Source: CAD feature listing. Evaluate the final solid. Frame: model axes, mm. A direction names the side the tool comes from. Round coordinates to 2 decimals unless told otherwise and drop trailing zeros. Write each loop counter-clockwise with the first axis right and the second up, starting at its lowest first coordinate (ties: lowest second). Pieces come first, ordered by that corner, then holes.
Autodesk Inventor part; units mm, degrees
ref_plane "YZ Plane" through (0, 0, 0) normal (1, 0, 0) x (0, 1, 0)
ref_plane "XZ Plane" through (0, 0, 0) normal (0, 1, 0) x (-1, 0, 0)
ref_plane "XY Plane" through (0, 0, 0) normal (0, 0, 1) x (1, 0, 0)
sketch "Sketch1" plane through (0, 0, 0) normal (0, 0, 1) x (1, 0, 0)
  line L0 (0, 0) -> (27, 0)
  line L1 (27, 0) -> (27, 10)
  line L2 (27, 10) -> (0, 10)
  line L3 (0, 10) -> (0, 0)
  line L4 (7.5, 0) -> (19.5, 0)
  line L5 (19.5, 0) -> (19.5, 5)
  line L6 (19.5, 5) -> (7.5, 5)
  line L7 (7.5, 5) -> (7.5, 0)
  point P0 (13.5, 5)
  point P1 (13.5, 10)
  dimension "d0" = 27
  dimension "d1" = 10
  dimension "d2" = 5
  dimension "d3" = 12
extrude "Extrusion1" add sketch "Sketch1" along normal blind 34.7 contours L3 L2 L1 L0 L5 L6 L7
chamfer "Chamfer1" distance 1 angle 45 2 edges at (27, 10, 17.35) (0, 10, 17.35)
chamfer "Chamfer2" distance 0.5 angle 45 2 edges at (7.5, 5, 17.35) (19.5, 5, 17.35)
sketch "Sketch2" plane through (1, 10, 0) normal (0, 1, 0) x (1, 0, 0)
  line L0 (18, -34.7) -> (18, 0)
  line L1 (-1, 0) -> (-1, -34.7)
  line L2 (25, 0) -> (0, 0)
  line L3 (5, -9.85) -> (20, -9.85)
  line L4 (20, -9.85) -> (20, -24.85)
  line L5 (20, -24.85) -> (5, -24.85)
  line L6 (5, -24.85) -> (5, -9.85)
  line L7 (25, 0) -> (25, -34.7)
  point P0 (-1, -17.35)
  point P1 (12.5, 0)
  point P2 (12.5, -9.85)
  point P3 (12.5, 0)
  point P4 (20, -17.35)
  point P5 (25, -17.35)
  dimension "d12" = 15
  dimension "d13" = 15
hole "Hole1" at (21, 10, 9.85) at (21, 10, 24.85) at (6, 10, 24.85) at (6, 10, 9.85) direction (0, -1, 0) diameter 3.242 depth 5 tip angle 118
sketch "Sketch3" plane through (0, 0, 34.7) normal (0, 0, 1) x (1, 0, 0)
  line L0 (0, 9) -> (0, 0)
  line L1 (0, 9) -> (1, 10)
  line L2 (26, 10) -> (1, 10)
  line L3 (26, 10) -> (27, 9)
  line L4 (27, 0) -> (27, 9)
  line L5 (0.375, 0) -> (0.375, 8.8447)
  line L6 (0.375, 8.8447) -> (1.1553, 9.625)
  line L7 (1.1553, 9.625) -> (25.8447, 9.625)
  line L8 (25.8447, 9.625) -> (26.625, 8.8447)
  line L9 (26.625, 8.8447) -> (26.625, 0)
  line L10 (19.5, 0) -> (27, 0)
  line L11 (26.625, 0) -> (27, 0)
  line L12 (27, 0) -> (0.375, 0)
  line L13 (0, 0) -> (7.5, 0)
  line L14 (0.375, 0) -> (0, 0)
  dimension "d21" = 0.375
extrude "Extrusion2" cut sketch "Sketch3" against normal blind 5 contours L1 L2 L3 L4 L10 L9 L8 L7 L6 L5 L13 L0
ref_plane "Work Plane1" through (0, 0, 17.35) normal (0, 0, 1) x (1, 0, 0)
mirror "Mirror1" about plane through (0, 0, 17.35) normal (0, 0, 1) of "Extrusion2"
sketch "Sketch4" plane through (1, 10, 29.7) normal (0, 1, 0) x (1, 0, 0)
  circle A0 centre (5, 19.85) radius 1.621
  circle A1 centre (20, 4.85) radius 1.621
  circle A2 centre (20, 19.85) radius 1.621
  circle A3 centre (5, 4.85) radius 1.621
  line L0 (25, 24.7) -> (0, 24.7)
  line L1 (0, 0) -> (0, 24.7)
  line L2 (0, 0) -> (25, 0)
  line L3 (25, 24.7) -> (25, 0)
  line L4 (25, 24.7) -> (0, 24.7)
  line L5 (0, 0) -> (25, 0)
  line L6 (9, 24.7) -> (16, 24.7)
  line L7 (16, 24.7) -> (16, 0)
  line L8 (16, 0) -> (9, 0)
  line L9 (9, 0) -> (9, 24.7)
  point P0 (-1, 29.7)
  point P1 (12.5, 24.7)
  point P2 (12.5, 24.7)
  dimension "d24" = 7
extrude "Extrusion3" cut sketch "Sketch4" against normal blind 0.35 contours L7 L2 L9 L0
properties part number "MGN Block"
1) Section query C-C on x = 15.25. Return the cut outline in (y, z) (3 decimals), then the cut area to 3 significant figures.
Taken from the geometry:
outline: (5, 0) - (9.625, 0) - (9.625, 5) - (9.65, 5) - (9.65, 29.7) - (9.625, 29.7) - (9.625, 34.7) - (5, 34.7) - close
area: 161 mm2
2) Section query A-A on y = 2.25. Return the cut outline in (x, z) (3 decimals).
Taken from the geometry:
outline: (0, 5) - (0.375, 5) - (0.375, 0) - (7.5, 0) - (7.5, 34.7) - (0.375, 34.7) - (0.375, 29.7) - (0, 29.7) - close; (19.5, 0) - (26.625, 0) - (26.625, 5) - (27, 5) - (27, 29.7) - (26.625, 29.7) - (26.625, 34.7) - (19.5, 34.7) - close
3) Material intervals for line 1 (Z direction, x = 6, y = 6.2); line 2 (X direction, y = 7.15, z = 9.85); line 3 (X direction, y = 4.5, z = 25), sorted ascending.
Taken from the geometry:
line 1: z = 0 to 8.23, 11.47 to 23.23, 26.47 to 34.7
line 2: x = 0 to 4.38, 7.62 to 19.38, 22.62 to 27
line 3: x = 0 to 5.23, 6.77 to 7.5, 19.5 to 20.23, 21.77 to 27
4) Section query B-B on z = 16. Return the cut outline in (x, y), then the cut area to 3 significant figures.
Taken from the geometry:
outline: (0, 0) - (7.5, 0) - (7.5, 4.5) - (8, 5) - (19, 5) - (19.5, 4.5) - (19.5, 0) - (27, 0) - (27, 9) - (26, 10) - (17, 10) - (17, 9.65) - (10, 9.65) - (10, 10) - (1, 10) - (0, 9) - close
area: 207 mm2
5) Contact query for flat-ended pins moving along their axis: P1, Ø1.5, axis at x = 18, z = 3, coming from the +Y side (3 decimals); P2, Ø5.5, axis at x = 16, z = 13.5, coming from the -Y side; P3, Ø2.5, axis at y = 4.5, z = 2.5, coming from the +X side (3 decimals). Output: stop coordinate, or through.
Taken from the geometry:
P1: stops at y = 9.625
P2: stops at y = 5
P3: stops at x = 26.625
6) Reachability of faces 4 (the face through (26.625, 4, 32)), 5 (the face through (14, 5, 17)), 6 (the face through (21.986, 7.465, 23.564)), 7 (the face through (14, 9.625, 2)), 8 (the face through (26.625, 4, 2)) from +Z, -Z, +X, -X, +Y, -Y: full face, straight path, thin tool, end or side. Return the list, or none.
Taken from the geometry:
face 4: +Z, +X, +Y, -Y
face 5: +Z, -Z, -Y
face 6: +Y
face 7: -Z, +X, -X, +Y
face 8: -Z, +X, +Y, -Y
7) Pull-direction query (Z, two-part tool) for faces 1 (the face through (13, 9.625, 32)), 2 (the face through (22.582, 7.465, 9.499)), 3 (the face through (17.4, 9.8, 29.7)); classes: released by +Z, released by -Z, zero draft, split by the parting line, or undercut.
Taken from the geometry:
face 1: zero draft
face 2: undercut
face 3: released by +Z
